Read the model definition and answer for the solid it produces. Units are mm, in the model's axes. A direction names the side the tool comes from. Coordinates: 2 decimals unless noted, no trailing zeros. Loops run counter-clockwise (first coordinate to the right, second up) from the corner with the lowest first, then second, coordinate; pieces in that order, holes last. Notation, with made-up numbers: (44.5, -19) - (89.5, -19) arc R19 cw to (89.5, -4) - close; hole circle Ø9 at (59.5, -32). An arc over 180 degrees is marked (long way). One line per question, with ' | ' between items. Start each with the question number.
Autodesk Fusion 360 part; units mm, degrees
sketch "Sketch1" plane through (0, 0, 0) normal (0, 0, 1) x (1, 0, 0)
  line L0 (0, 0) -> (0, 300.4312) construction
  circle A0 centre (0, 300.4312) radius 12.7
  line L1 (25.4, 0) -> (-25.4, 0)
  line L2 (-25.4, 0) -> (-25.4, 330.2)
  line L3 (-25.4, 330.2) -> (25.4, 330.2)
  line L4 (25.4, 330.2) -> (25.4, 0)
  dimension "d1" = 300.4312
  dimension "d2" = 25.4
  dimension "d3" = 50.8
  dimension "d4" = 330.2
extrude "Extrude1" add sketch "Sketch1" along normal blind 25.4 contours A0 | L1 L2 L3 L4
sketch "Sketch2" plane through (0, 330.2, 0) normal (0, 1, 0) x (-1, 0, 0)
  line L0 (-25.4, 0) -> (25.4, 0)
  line L1 (25.4, 0) -> (25.4, 25.4)
  line L2 (25.4, 25.4) -> (-25.4, 25.4)
  line L3 (-25.4, 25.4) -> (-25.4, 0)
  line L4 (-22.225, 22.225) -> (-22.225, 3.175)
  line L5 (-22.225, 3.175) -> (22.225, 3.175)
  line L6 (22.225, 3.175) -> (22.225, 22.225)
  line L7 (22.225, 22.225) -> (-22.225, 22.225)
  dimension "d7" = -3.175
extrude "Extrude2" cut sketch "Sketch2" against normal up to surface (330.2 mm away) contours L4 L5 L6 L7
extrude "Extrude3" cut sketch "Sketch1" along normal blind 3.175 contours A0
move_face "OffsetFaces1" offset -43.4594 1 faces at (7.4083, 0, 1.0583)
sketch "Sketch3" plane through (0, 0, 0) normal (0, 0, 1) x (1, 0, 0)
  line L0 (-12.7, 300.4312) -> (-6.35, 289.4327) construction
  line L1 (-6.35, 289.4327) -> (6.35, 289.4327) construction
  line L2 (6.35, 289.4327) -> (12.7, 300.4312) construction
  line L3 (12.7, 300.4312) -> (6.35, 311.4297) construction
  line L4 (6.35, 311.4297) -> (-6.35, 311.4297) construction
  line L5 (-6.35, 311.4297) -> (-12.7, 300.4312) construction
  circle A0 centre (0, 300.4312) radius 30.48 construction
  circle A1 centre (0, 239.4712) radius 30.48 construction
  circle A2 centre (0, 239.4712) radius 14.2748
  point P0 (0, 300.4312)
  dimension "d19" = 12.7
  dimension "d20" = 60.96
  dimension "d21" = 60.96
  dimension "d22" = 28.5496
extrude "Extrude5" cut sketch "Sketch3" along normal blind 50.8
component "Intake Support" placed x (1, 0, 0) y (0, 1, 0) z (0, 0, 1) at (0, 0, 0)
equation "d12 = -3 in + 1.289 in"
1) Which of the six approach directions +Z, -Z, +X, -X, +Y, -Y give full straight-line access (tool end or side, diameter ignored) to faces 1 (the flat face through (0, 189, 25.4)), 2 (the flat face through (0, 189, 22.225)), 3 (the cylindrical face through (-2.75, 312.83, 1.57))?
2) Given pin 1 Ø23 at (x, y) = (0, 239.47) entering from +Z; pin 2 Ø13.5 at (x, y) = (-9, 165) entering from -Z, each flat-ended and moving along its own axis, determine where each tip first touches the part or whether it passes through.
3) The part is cut by section D-D on y = 244.5. Write down the section's boundary in (x, z) (3 decimals), and give its area (3 significant figures).
4) The part is cut by section C-C on x = 0. Write down the section's boundary in (y, z) (3 decimals).
5) Find the intervals of material crossed by line 1 along Y through (x, z) = (0, 1.6); line 2 along Z through (x, y) = (-5.5, 263.5) (3 decimals); line 3 along Y through (x, z) = (0, 23.2), in increasing order. Write a range as from..to.
6) The part is cut by section B-B on x = -18. Write down the section's boundary in (y, z) (3 decimals).
7) The part is cut by section A-A on z = 18.75. Write down the section's boundary in (x, y) (3 decimals).
8) The mould has two halves that part along X. Classify faces 4 (the flat face through (-22.225, 189, 13)), 5 (the flat face through (-25.4, 185, 13)), 6 (the cylindrical face through (-3.094, 253.407, 1.565)), 7 (the flat face through (0, 43.459, 2)): released by +X, released by -X, zero draft, split by the parting line, or undercut.
Answer below:
1) face 1: +Z, +X, -X, +Y, -Y | face 2: +Y, -Y | face 3: -Z
2) pin 1: through | pin 2: z = 0
3) outline: (-25.4, 0) - (-13.36, 0) - (-13.36, 3.175) - (-22.225, 3.175) - (-22.225, 22.225) - (-13.36, 22.225) - (-13.36, 25.4) - (-25.4, 25.4) - close; (13.36, 0) - (25.4, 0) - (25.4, 25.4) - (13.36, 25.4) - (13.36, 22.225) - (22.225, 22.225) - (22.225, 3.175) - (13.36, 3.175) - close | area: 274 mm2
4) outline: (43.459, 0) - (225.196, 0) - (225.196, 3.175) - (43.459, 3.175) - close; (43.459, 22.225) - (225.196, 22.225) - (225.196, 25.4) - (43.459, 25.4) - close; (253.746, 0) - (287.731, 0) - (287.731, 3.175) - (253.746, 3.175) - close; (253.746, 22.225) - (330.2, 22.225) - (330.2, 25.4) - (253.746, 25.4) - close; (313.131, 0) - (330.2, 0) - (330.2, 3.175) - (313.131, 3.175) - close
5) line 1: 43.46..225.2, 253.75..287.73, 313.13..330.2 | line 2: 0..3.175, 22.225..25.4 | line 3: 43.46..225.2, 253.75..330.2
6) outline: (43.459, 0) - (330.2, 0) - (330.2, 3.175) - (43.459, 3.175) - close; (43.459, 22.225) - (330.2, 22.225) - (330.2, 25.4) - (43.459, 25.4) - close
7) outline: (-25.4, 43.459) - (-22.225, 43.459) - (-22.225, 330.2) - (-25.4, 330.2) - close; (22.225, 43.459) - (25.4, 43.459) - (25.4, 330.2) - (22.225, 330.2) - close
8) face 4: undercut | face 5: released by -X | face 6: undercut | face 7: zero draft
